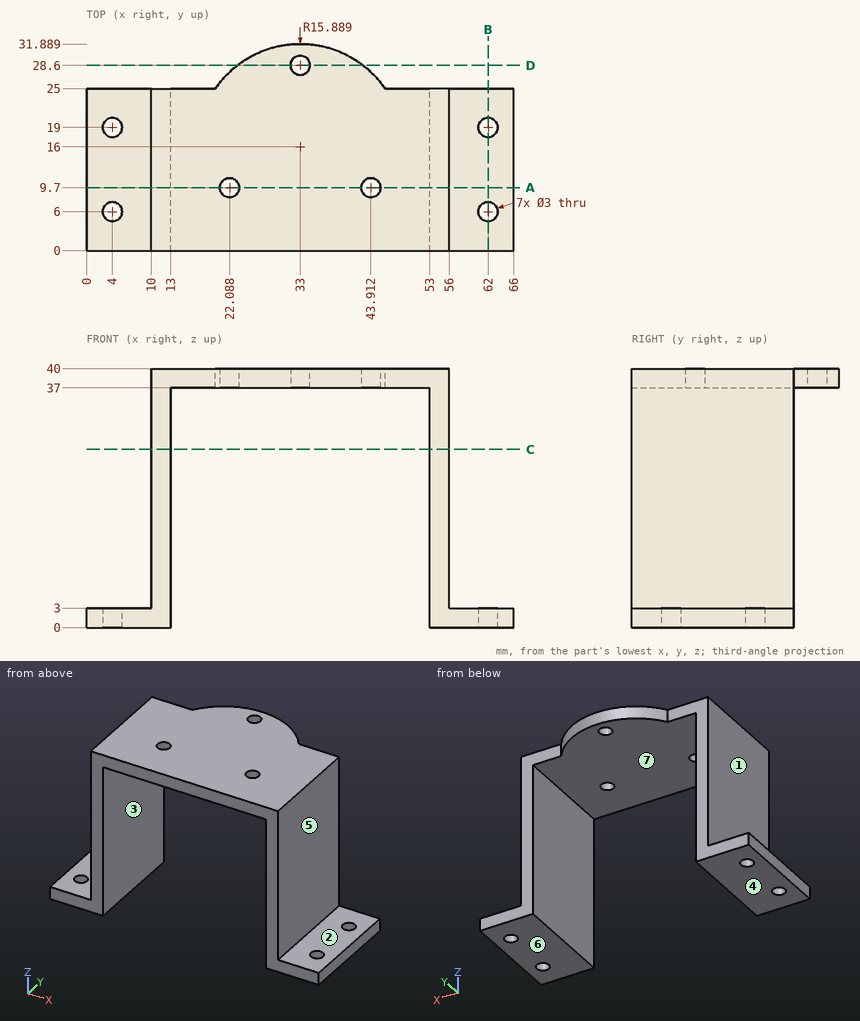
Study the drawing (mm; zero at the part's minimum x, y, z) and answer. A direction names the side the tool comes from. Round coordinates to 2 decimals unless told otherwise and drop trailing zeros. Write each loop counter-clockwise with the first axis right and the second up, starting at its lowest first coordinate (ties: lowest second). Pieces come first, ordered by that corner, then holes.
1) Determine the mould class of the marked faces 5, 6 and 7 for opening direction X: pulls with the +X half, pulls with the -X half, needs draft (parallel to the pull), parting line crosses it, or undercut.
2) Flat-ended cylindrical pins translate along their axes: P1, Ø12.5, axis at y = 11, z = 23, coming from the +X side; P2, Ø4, axis at y = 21.5, z = 6, coming from the -X side; P3, Ø3, axis at x = 59.5, y = 8.5, coming from the +Z side; P4, Ø1.8, axis at x = 62, y = 6, coming from the +Z side. Find the tip coordinate at first contact, or state that the pin passes through.
3) A cutting plane is placed at D-D on y = 28.6. Determine the outline of the cut face in (x, z).
4) A cutting plane is placed at C-C on z = 27.5. Determine the outline of the cut face in (x, y).
5) A cutting plane is placed at B-B on x = 62. Determine the outline of the cut face in (y, z), and give its area (3 significant figures).
6) Which of the six approach directions +Z, -Z, +X, -X, +Y, -Y give full straight-line access (tool end or side, diameter ignored) to the marked faces 1, 2, 3 and 4?
7) Consider probe 1 along Y at (x, z) = (4, 1.8); probe 2 along X at (y, z) = (19, 1.95); probe 3 along X at (y, z) = (17.5, 6.5). Determine where each line is inside the solid, lowest interval first.
8) A cutting plane is placed at A-A on y = 9.7. Determine the outline of the cut face in (x, z).
Entries:
1. face 5: pulls with the +X half
1. face 6: needs draft
1. face 7: undercut
2. P1: stops at x = 56
2. P2: stops at x = 10
2. P3: stops at z = 3
2. P4: passes through
3. outline: (23.32, 37) - (31.5, 37) - (31.5, 40) - (23.32, 40) - close; (34.5, 37) - (42.68, 37) - (42.68, 40) - (34.5, 40) - close
4. outline: (10, 0) - (13, 0) - (13, 25) - (10, 25) - close; (53, 0) - (56, 0) - (56, 25) - (53, 25) - close
5. outline: (0, 0) - (4.5, 0) - (4.5, 3) - (0, 3) - close; (7.5, 0) - (17.5, 0) - (17.5, 3) - (7.5, 3) - close; (20.5, 0) - (25, 0) - (25, 3) - (20.5, 3) - close
5. area: 57.0 mm2
6. face 1: +Z, -X, +Y, -Y
6. face 2: +Z, +X, +Y, -Y
6. face 3: -Z, +Y, -Y
6. face 4: -Z, +X, -X, +Y, -Y
7. probe 1: y = 0 to 4.5, 7.5 to 17.5, 20.5 to 25
7. probe 2: x = 0 to 2.5, 5.5 to 13, 53 to 60.5, 63.5 to 66
7. probe 3: x = 10 to 13, 53 to 56
8. outline: (0, 0) - (13, 0) - (13, 37) - (20.59, 37) - (20.59, 40) - (10, 40) - (10, 3) - (0, 3) - close; (23.59, 37) - (42.41, 37) - (42.41, 40) - (23.59, 40) - close; (45.41, 37) - (53, 37) - (53, 0) - (66, 0) - (66, 3) - (56, 3) - (56, 40) - (45.41, 40) - close
